The model under review builds one solid part; all positions refer to its coordinate system, in mm. A direction names the side the tool comes from. Round coordinates to 2 decimals unless told otherwise and drop trailing zeros. Order: outer loops, then holes, each group sorted by start corner. A loop starts at its lowest first (then second) coordinate and runs counter-clockwise, first axis right, second up. Notation, with made-up numbers: (24, -9.5) -> (46, -9.5) arc R17 ccw to (46, 1.5) -> close; hole circle Ø1 at (51.5, 18.25). An arc over 180 degrees is marked (long way). Put each result on its own line as item: value. Start each with the question number.
from build123d import *

# Parameters (mm, degrees)
F1_DEPTH = 5.715
F2_DEPTH = 3.175
F3_R     = 1.27
F4_DEPTH = 25.4


with BuildPart() as f1:
    # F0 (on Front) → F1 (new body, symmetric)
    with BuildSketch(Plane.XZ):
        with BuildLine():
            ThreePointArc((9.215210569, -2.4094644982), (9.4472351953, -1.2146489884), (9.525, 0))
            ThreePointArc((9.525, 0), (9.4472351953, 1.2146489884), (9.215210569, 2.4094644982))
            Line((9.215210569, 2.4094644982), (9.215210569, -2.4094644982))
        make_face()
        with BuildLine():
            Line((9.215210569, -2.4094644982), (9.215210569, 2.4094644982))
            ThreePointArc((9.215210569, 2.4094644982), (-9.525, 0), (9.215210569, -2.4094644982))
        make_face()
    extrude(amount=F1_DEPTH, both=True)

    # F0 (on Front) → F2 (join, symmetric)
    with BuildSketch(Plane.XZ):
        with BuildLine():
            ThreePointArc((9.215210569, 2.4094644982), (9.4472351953, 1.2146489884), (9.525, 0))
            ThreePointArc((9.525, 0), (9.4472351953, -1.2146489884), (9.215210569, -2.4094644982))
            Line((9.215210569, -2.4094644982), (9.215210569, -2.6859357022))
            Line((9.215210569, -2.6859357022), (49.855210569, -2.6859357022))
            Line((49.855210569, -2.6859357022), (49.855210569, 2.4094644982))
            Line((49.855210569, 2.4094644982), (9.215210569, 2.4094644982))
        make_face()
        Polygon((71.9085857272, -19.0247967839), (49.855210569, 2.4094644982), (49.855210569, -2.6859357022), (69.9069363303, -23.3931405965), (100.4668754262, -23.3931405965), (97.190618515, -19.0247967839), align=None)
    extrude(amount=F2_DEPTH, both=True)

    # F3 (on face) → F4 (cut)
    with BuildSketch(Plane.XZ.offset(5.715)):
        Circle(F3_R)
    extrude(amount=-F4_DEPTH, mode=Mode.SUBTRACT)


solid = f1.part
Q1. Clearance check with flat-ended pins moving along their axes: pin 1 Ø3 at (x, y) = (79.5, 0) entering from +Z; pin 2 Ø1.5 at (x, y) = (66.5, -1.5) entering from -Z; pin 3 Ø10 at (x, z) = (37, 3) entering from -Y (3 decimals); pin 4 Ø5 at (y, z) = (-3, -1.5) entering from -X (3 decimals). State where each tip first meets the part, or that it passes through.
Q2. For faces 1 (the face through (30, 0, 2.409)), 2 (the face through (29, 0, -2.686)), 3 (the face through (55, -3.175, -7)), 4 (the face through (55, 3.175, -7)), list the 3-axis set-ups (+Z, -Z, +X, -X, +Y, -Y) from which the entire face can be reached by the end or side of a thin tool; tool diameter is ignored.
Q3. Wall thickness on probe 1 along Z at (x, y) = (0, -0.5) (3 decimals); probe 2 along Z at (x, y) = (47.5, -0.5); probe 3 along Z at (x, y) = (92, 1): over which ranges is each line inside the solid? List them lowest first. Write a range as [from, to].
Q4. Draft analysis for pull direction X (two halves, no side actions). For faces 5 (the face through (0, -5.715, -2)), 6 (the face through (98.85, -0.04, -21.24)), 7 (the face through (-0.17, -0.08, 1.26)), state which applies: +X half, -X half, draft (parallel to the pull), parting line (faces both ways), or undercut.
Q5. Take a section at C-C on x = 88.5. Give the boundary of the cut face in (y, z) (3 decimals), and give its area (3 significant figures).
Q6. Take a section at D-D on z = 4.5. Give the boundary of the cut face in (x, y) (3 decimals), and give its area (3 significant figures).
Q7. Take a section at A-A on x = 0. Give the boundary of the cut face in (y, z) (3 decimals).
Q8. Take a section at B-B on y = 4.25. Give the boundary of the cut face in (x, z) (3 decimals).
Calculated:
1. pin 1: stops at z = -19.02
1. pin 2: stops at z = -20.65
1. pin 3: stops at y = -3.175
1. pin 4: stops at x = -9.525
2. face 1: +Z, +X, +Y, -Y
2. face 2: -Z, +Y, -Y
2. face 3: +Z, -Z, +X, -Y
2. face 4: +Z, -Z, +X, +Y
3. probe 1: z = [-9.525, -1.27], [1.27, 9.525]
3. probe 2: z = [-2.69, 2.41]
3. probe 3: z = [-23.39, -19.02]
4. face 5: draft
4. face 6: +X half
4. face 7: undercut
5. outline: (-3.175, -23.393) -> (3.175, -23.393) -> (3.175, -19.025) -> (-3.175, -19.025) -> close
5. area: 27.7 mm²
6. outline: (-8.395, -5.715) -> (8.395, -5.715) -> (8.395, 5.715) -> (-8.395, 5.715) -> close
6. area: 192 mm²
7. outline: (-5.715, -9.525) -> (5.715, -9.525) -> (5.715, -1.27) -> (-5.715, -1.27) -> close; (-5.715, 1.27) -> (5.715, 1.27) -> (5.715, 9.525) -> (-5.715, 9.525) -> close
8. outline: circle Ø19.05 at (0, 0); hole circle Ø2.54 at (0, 0)
